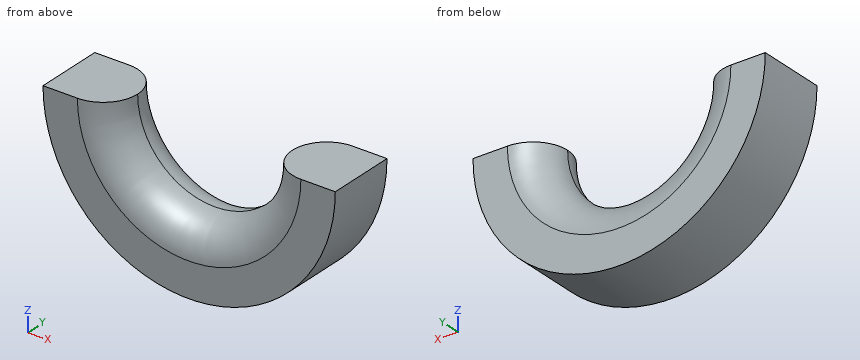
from build123d import *

# Parameters (mm, degrees)
BOSS_EXTRUDE1_DEPTH = 2
FILLET1_R           = 1


with BuildPart() as part:
    # Sketch1 → Boss-Extrude1 (new body)
    with BuildSketch(Plane(origin=(0, 0, 0), x_dir=(1, 0, 0), z_dir=(0, 1, 0))):
        with BuildLine():
            Line((-4.25, 0), (-2.25, 0))
            ThreePointArc((-2.25, 0), (0, 2.25), (2.25, 0))
            Line((2.25, 0), (4.25, 0))
            ThreePointArc((4.25, 0), (0, 4.25), (-4.25, 0))
        make_face()
    extrude(amount=BOSS_EXTRUDE1_DEPTH)

    # Fillet1
    fillet1_edges = [part.edges().sort_by_distance(p)[0] for p in [
        (0, 0, -2.25),
        (0, 2, -2.25),
    ]]
    fillet(fillet1_edges, radius=FILLET1_R - 0.0001)  # a hair under: the kernel refuses the full size


solid = part.part
Could you check a few things on this model? Use its own coordinates, in mm. Give positions to 0.01 mm unless a question says otherwise; leave off trailing zeros. Order: outer loops, then holes, each group sorted by start corner. A loop starts at its lowest first (then second) coordinate and runs counter-clockwise, first axis right, second up.
1. Suppose I cut it at C-C (y = 1.25). Write out the boundary of the cut face in (x, z).
Answers below:
outline: (-4.25, 0) arc R4.25 ccw to (4.25, 0) - (2.28, 0) arc R2.28 cw to (-2.28, 0) - close
2. I need wall thicknesses on L1, parallel to X at y = 0.25, z = -0.3; L2, parallel to X at y = 0.6, z = -0.8; L3, parallel to X at y = 0.55, z = -2.5. Which ranges of each line are inside material? Lowest first, please.
Answers below:
L1: x = -4.24 to -2.57, 2.57 to 4.24
L2: x = -4.17 to -2.19, 2.19 to 4.17
L3: x = -3.44 to 3.44
3. Suppose I cut it at B-B (z = -3.4). Write out the boundary of the cut face in (x, y), plus the area to 3 significant figures.
Answers below:
outline: (-2.55, 0) - (2.55, 0) - (2.55, 2) - (-2.55, 2) - close
area: 10.2 mm2
4. For pin 1 (1 mm diameter, centred on x = 2, y = 1, fed in from -Z), with a flat end and sliding along its axis, tell me the tip position at first contact or that it passes through.
Answers below:
pin 1: stops at z = -3.98
